CAD build for the part. Positions are in the model's coordinates, mm. A direction names the side the tool comes from. Give positions to 0.01 mm unless a question says otherwise; leave off trailing zeros. Order: outer loops, then holes, each group sorted by start corner. A loop starts at its lowest first (then second) coordinate and runs counter-clockwise, first axis right, second up. Notation, with made-up numbers: M 51,-39 L 63,-39 A19 cw 63,-8 Z; hole C -28.75,-13 d11. An arc over 180 degrees is marked long. Put each result on its own line as item: value. Start each with the question number.
1) Two-plate mould, pull along Z, no slides. Class faces 1 (the face through (-16.986, -4.444, 20.013)), 2 (the face through (-18, 6, -20)), 3 (the face through (-8, 44, 0)): released by +Z, released by -Z, zero draft, split by the parting line, or undercut.
2) Pin check, flat tips, straight feed: pin 1 (13.5 mm diameter, centred on y = 36, z = 0, fed in from +X); pin 2 (4 mm diameter, centred on x = -4, y = 22.5, fed in from -Z); pin 3 (10 mm diameter, centred on x = -12, y = 9, fed in from -Z); pin 4 (15 mm diameter, centred on y = 3.5, z = -9.5, fed in from +X). Stop position of each tip, or through.
3) Drill centre lines: line 1 (Y direction, x = -4.25, z = 0); line 2 (Y direction, x = -3.25, z = 5); line 3 (X direction, y = 16.5, z = 22). Where is each one in solid material? Low to high. Write a range as [from, to].
4) Cut at A-A (y = -36). Write the cut outline in (x, z), and give its area (3 significant figures).
5) Cut at D-D (y = 0). Give the number of separate pieces and of enclosed holes in the cut face, and give its area (3 significant figures).
6) Tool access for faces 4 (the face through (-9.9, 22.4, -7.1)), 5 (the face through (-12.352, 40.214, -0.553)), 6 (the face through (-17.16, -5.85, 26.36)): list every direction of +Z, -Z, +X, -X, +Y, -Y with a clear straight run to the whole face (end or side of a thin tool).
7) Cut at B-B (x = -7). Write the cut outline in (y, z), and give its area (3 significant figures).
8) Cut at C-C (z = 34.5). Write the cut outline in (x, y), and give its area (3 significant figures).
```python
from build123d import *

# Parameters (mm, degrees)
FILLET1_R            = 0.3
DIAMETER_HOLE1_D     = 14
DIAMETER_HOLE1_DEPTH = 8.6
TAPPED_HOLE1_D       = 8.5
CUT_EXTRUDE1_DEPTH   = 65.249513617


with BuildPart() as part:
    # Sketch1 → Revolve1 (revolve)
    with BuildSketch(Plane.XY):
        Polygon((0, 44), (-16, 44), (-16, 27), (-18, 27), (-18, 20.5), (-16, 20.5), (-16, 23.5), (-4, 23.5), (-4, 24.75), (-2.1, 24.75), (-2.1, 23.5), (0, 23.5), align=None)
    revolve(axis=Axis((0, 0, 0), (-1, 0, 0)))

    # Fillet1
    fillet1_edges = [part.edges().sort_by_distance(p)[0] for p in [
        (-16, -27, 0),
    ]]
    fillet(fillet1_edges, radius=FILLET1_R)

    # Diameter Hole1
    with Locations(Plane(origin=(0, 0, 0), x_dir=(0, 0, -1), z_dir=(1, 0, 0))):
        with Locations((0, 36), (-36, 0), (36, 0), (0, -36)):
            Hole(DIAMETER_HOLE1_D / 2, depth=DIAMETER_HOLE1_DEPTH)

    # Tapped Hole1 (through all)
    with Locations(Plane(origin=(-8.6, 0, 0), x_dir=(0, 0, -1), z_dir=(1, 0, 0))):
        with Locations((0, 36), (-36, 0), (0, -36), (36, 0)):
            Hole(TAPPED_HOLE1_D / 2)

    # Sketch6 → Cut-Extrude1 (cut, through all)
    with BuildSketch(Plane(origin=(-16, 0, 0), x_dir=(0, 0, -1), z_dir=(1, 0, 0))):
        with BuildLine():
            Line((-43.859219924, 3.516934416), (-3.516934416, 43.859219924))
            ThreePointArc((-3.516934416, 43.859219924), (-31.112698372, 31.112698372), (-43.859219924, 3.516934416))
        make_face()
        with BuildLine():
            Line((3.516934416, 43.859219924), (43.859219924, 3.516934416))
            ThreePointArc((43.859219924, 3.516934416), (31.112698372, 31.112698372), (3.516934416, 43.859219924))
        make_face()
        with BuildLine():
            Line((43.859219924, -3.516934416), (3.516934416, -43.859219924))
            ThreePointArc((3.516934416, -43.859219924), (31.112698372, -31.112698372), (43.859219924, -3.516934416))
        make_face()
        with BuildLine():
            Line((-3.516934416, -43.859219924), (-43.859219924, -3.516934416))
            ThreePointArc((-43.859219924, -3.516934416), (-31.112698372, -31.112698372), (-3.516934416, -43.859219924))
        make_face()
    extrude(amount=CUT_EXTRUDE1_DEPTH, mode=Mode.SUBTRACT)


solid = part.part
```
Solution:
1. face 1: undercut
1. face 2: zero draft
1. face 3: split by the parting line
2. pin 1: x = -8.6
2. pin 2: z = -26.88
2. pin 3: z = -43.38
2. pin 4: through
3. line 1: [-44, -43], [-29, -23.5], [23.5, 29], [43, 44]
3. line 2: [-42.38, -40.9], [-31.1, -24.24], [24.24, 31.1], [40.9, 42.38]
3. line 3: [-16, 0]
4. outline: M -16,-11.38 L 0,-11.38 L 0,-7 L -8.6,-7 L -8.6,-4.25 L -16,-4.25 Z; M -16,4.25 L -8.6,4.25 L -8.6,7 L 0,7 L 0,11.38 L -16,11.38 Z
4. area: 181 mm²
5. separate pieces: 4
5. enclosed holes: 0
5. area: 311 mm²
6. face 4: +X
6. face 5: +X, -X
6. face 6: -X
7. outline: M -43.86,-3.52 L -3.52,-43.86 A44 ccw 3.52,-43.86 L 43.86,-3.52 A44 ccw 43.86,3.52 L 3.52,43.86 A44 ccw -3.52,43.86 L -43.86,3.52 A44 ccw Z; hole C -36,0 d14; hole C 0,0 d47; hole C 0,-36 d14; hole C 0,36 d14; hole C 36,0 d14
7. area: 2,090 mm²
8. outline: M -16,-12.88 L 0,-12.88 L 0,-6.84 L -8.6,-6.84 L -8.6,-3.98 L -16,-3.98 Z; M -16,3.98 L -8.6,3.98 L -8.6,6.84 L 0,6.84 L 0,12.88 L -16,12.88 Z
8. area: 236 mm²
